Work out the finished part from the listing and answer in its coordinate system (mm). Give positions to 0.01 mm unless a question says otherwise; leave off trailing zeros. Loops run counter-clockwise (first coordinate to the right, second up) from the corner with the lowest first, then second, coordinate; pieces in that order, holes last. Notation, with made-up numbers: (26, -28) -> (61, -28) arc R10 cw to (61, -22) -> close; hole circle Ø6 at (7, 47). An arc over 180 degrees is marked (long way). Answer as CSV lines item,"result". Start each with the question number.
1. Find section D-D, the plane x = 15. Give the vertices of the cut face in (y, z).
2. Find the intervals of material crossed by line 1 along Z through (x, y) = (14.5, 2.5); line 2 along X through (y, z) = (6, 1); line 3 along X through (y, z) = (8.65, 72.5), in increasing order.
3. Find section C-C, the plane x = -7.5. Give the vertices of the cut face in (y, z), and give its area (3 significant figures).
4. Find section B-B, the plane y = 9.25. Give the vertices of the cut face in (x, z), and give its area (3 significant figures).
5. A flat-ended cylindrical pin translates along its axis: pin 1 Ø5 at (x, z) = (15, -72.5) entering from -Y. Find the tip coordinate at first contact, or state that the pin passes through.
6. Find section A-A, the plane z = -50. Give the vertices of the cut face in (x, y), and give its area (3 significant figures).
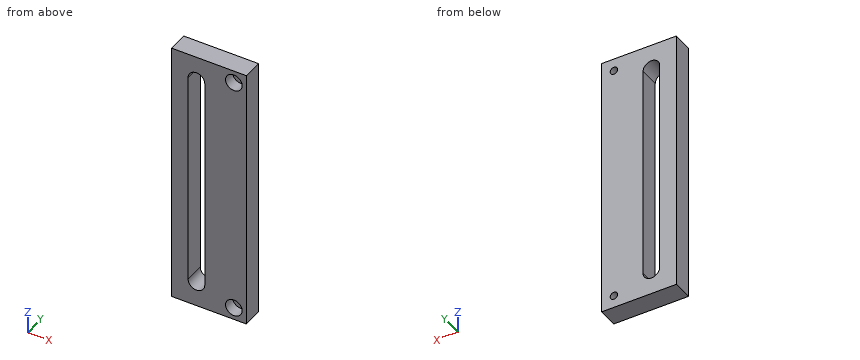
from build123d import *

# Parameters (mm, degrees)
SKETCH2_W           = 45
SKETCH2_H           = 160
BOSS_EXTRUDE3_DEPTH = 12
SKETCH3_R           = 2.25
CUT_EXTRUDE3_DEPTH  = 5
SKETCH5_R           = 5
CUT_EXTRUDE5_DEPTH  = 7
CUT_EXTRUDE6_DEPTH  = 84.965766834


with BuildPart() as part:
    # Sketch2 → Boss-Extrude3 (new body)
    with BuildSketch(Plane(origin=(0, 0, 0), x_dir=(1, 0, 0), z_dir=(0, 1, 0))):
        Rectangle(SKETCH2_W, SKETCH2_H)
    extrude(amount=BOSS_EXTRUDE3_DEPTH)

    # Sketch3 → Cut-Extrude3 (cut)
    with BuildSketch(Plane(origin=(0, 12, 0), x_dir=(1, 0, 0), z_dir=(0, 1, 0))):
        with Locations(Location((15, 72.5, 0), (0, 0, 270))):
            Circle(SKETCH3_R)
        with Locations(Location((15, -72.5, 0), (0, 0, 270))):
            Circle(SKETCH3_R)
    cut_extrude3 = extrude(amount=-CUT_EXTRUDE3_DEPTH, mode=Mode.SUBTRACT)

    # Sketch5 → Cut-Extrude5 (cut)
    with BuildSketch(Plane(origin=(0, 7, 0), x_dir=(1, 0, 0), z_dir=(0, 1, 0))):
        with Locations(Location((15, 72.5, 0), (0, 0, 270))):
            Circle(SKETCH5_R)
    cut_extrude5 = extrude(amount=-CUT_EXTRUDE5_DEPTH, mode=Mode.SUBTRACT)

    # Mirror1: Cut-Extrude3, Cut-Extrude5 across plane
    add(cut_extrude3.mirror(Plane.XY), mode=Mode.SUBTRACT)
    add(cut_extrude5.mirror(Plane.XY), mode=Mode.SUBTRACT)

    # Sketch6 → Cut-Extrude6 (cut, through all)
    with BuildSketch(Plane(origin=(0, 12, 0), x_dir=(1, 0, 0), z_dir=(0, 1, 0))):
        with BuildLine():
            Line((-12.5, -65), (-12.5, 65))
            ThreePointArc((-12.5, 65), (-7.5, 70), (-2.5, 65))
            Line((-2.5, 65), (-2.5, -65))
            ThreePointArc((-2.5, -65), (-7.5, -70), (-12.5, -65))
        make_face()
    extrude(amount=-CUT_EXTRUDE6_DEPTH, mode=Mode.SUBTRACT)


solid = part.part
Resolved:
1,outline,"(0, -80) -> (12, -80) -> (12, -74.75) -> (7, -74.75) -> (7, -77.5) -> (0, -77.5) -> close; (0, -67.5) -> (7, -67.5) -> (7, -70.25) -> (12, -70.25) -> (12, 70.25) -> (7, 70.25) -> (7, 67.5) -> (0, 67.5) -> close; (0, 77.5) -> (7, 77.5) -> (7, 74.75) -> (12, 74.75) -> (12, 80) -> (0, 80) -> close"
2,line 1,"z = -80 to -77.47, -67.53 to 67.53, 77.47 to 80"
2,line 2,"x = -22.5 to -12.5, -2.5 to 22.5"
2,line 3,"x = -22.5 to 12.75, 17.25 to 22.5"
3,outline,"(0, -80) -> (12, -80) -> (12, -70) -> (0, -70) -> close; (0, 70) -> (12, 70) -> (12, 80) -> (0, 80) -> close"
3,area,"240 mm^2"
4,outline,"(-22.5, -80) -> (22.5, -80) -> (22.5, 80) -> (-22.5, 80) -> close; hole (-12.5, -65) arc R5 ccw to (-2.5, -65) -> (-2.5, 65) arc R5 ccw to (-12.5, 65) -> close; hole circle Ø4.5 at (15, -72.5); hole circle Ø4.5 at (15, 72.5)"
4,area,"5,790 mm^2"
5,pin 1,"stops at y = 7"
6,outline,"(-22.5, 0) -> (-12.5, 0) -> (-12.5, 12) -> (-22.5, 12) -> close; (-2.5, 0) -> (22.5, 0) -> (22.5, 12) -> (-2.5, 12) -> close"
6,area,"420 mm^2"
